Model file for the job. Use its own axes, mm. A direction names the side the tool comes from. Round coordinates to 2 decimals unless told otherwise and drop trailing zeros. Order: outer loops, then holes, each group sorted by start corner. A loop starts at its lowest first (then second) coordinate and runs counter-clockwise, first axis right, second up. Notation, with made-up numbers: (55, -33.5) - (59, -33.5) arc R13 cw to (59, -28.5) - close; hole circle Ø3 at (-30, -29). An arc over 180 degrees is marked (long way). Write item = value, one per line.
```python
from build123d import *

# Parameters (mm, degrees)
BOSS_EXTRUDE1_DEPTH                           = 2.54
CHAMFER1_SIZE                                 = 2.54
CSK_FOR_4_FLAT_HEAD_MACHINE_SCREW1_AT_2_COUNT = 2
CSK_FOR_4_FLAT_HEAD_MACHINE_SCREW1_AT_2_PITCH = 69.85
CSK_FOR_4_FLAT_HEAD_MACHINE_SCREW1_AT_3_COUNT = 2
CSK_FOR_4_FLAT_HEAD_MACHINE_SCREW1_AT_3_PITCH = 69.85
CSK_FOR_4_FLAT_HEAD_MACHINE_SCREW1_AT_4_COUNT = 2
CSK_FOR_4_FLAT_HEAD_MACHINE_SCREW1_AT_4_PITCH = 98.782817332
CUT_EXTRUDE2_DEPTH                            = 0.508


with BuildPart() as part:
    # Sketch1 → Boss-Extrude1 (new body)
    with BuildSketch(Plane(origin=(0, 0, 0), x_dir=(1, 0, 0), z_dir=(0, 1, 0))):
        with BuildLine():
            Line((-43.688, 34.925), (-43.688, -34.925))
            ThreePointArc((-43.688, -34.925), (-41.121376724, -41.121376724), (-34.925, -43.688))
            Line((-34.925, -43.688), (34.925, -43.688))
            ThreePointArc((34.925, -43.688), (41.121376724, -41.121376724), (43.688, -34.925))
            Line((43.688, -34.925), (43.688, 34.925))
            ThreePointArc((43.688, 34.925), (41.121376724, 41.121376724), (34.925, 43.688))
            Line((34.925, 43.688), (-34.925, 43.688))
            ThreePointArc((-34.925, 43.688), (-41.121376724, 41.121376724), (-43.688, 34.925))
        make_face()
    extrude(amount=BOSS_EXTRUDE1_DEPTH)

    # Chamfer1
    chamfer1_edges = [part.edges().sort_by_distance(p)[0] for p in [
        (-43.688, 0, 0),
        (-41.121376724, 0, 41.121376724),
        (-41.121376724, 0, -41.121376724),
        (0, 0, 43.688),
        (0, 0, -43.688),
        (41.121376724, 0, 41.121376724),
        (41.121376724, 0, -41.121376724),
        (43.688, 0, 0),
    ]]
    chamfer(chamfer1_edges, length=CHAMFER1_SIZE - 0.0001)  # a hair under: the kernel refuses the full size

    # Sketch6 → CSK for #4 Flat Head Machine Screw1 (revolve, cut)
    with BuildSketch(Plane(origin=(-34.925, 2.54, -34.925), x_dir=(0, 0, 1), z_dir=(1, 0, 0))):
        Polygon((0, 0), (0, 2.54), (1.7272, 2.54), (1.7272, 1.554265286), (3.0783022, 0), align=None)
    csk_for_4_flat_head_machine_screw1 = revolve(axis=Axis((-34.925, 8.89, -34.925), (0, -1, 0)), mode=Mode.SUBTRACT)

    # CSK for #4 Flat Head Machine Screw1 at 2: CSK for #4 Flat Head Machine Screw1 ×2
    with Locations(*[(i * CSK_FOR_4_FLAT_HEAD_MACHINE_SCREW1_AT_2_PITCH, 0, 0) for i in range(1, CSK_FOR_4_FLAT_HEAD_MACHINE_SCREW1_AT_2_COUNT)]):
        add(csk_for_4_flat_head_machine_screw1, mode=Mode.SUBTRACT)

    # CSK for #4 Flat Head Machine Screw1 at 3: CSK for #4 Flat Head Machine Screw1 ×2
    with Locations(*[(0, 0, i * CSK_FOR_4_FLAT_HEAD_MACHINE_SCREW1_AT_3_PITCH) for i in range(1, CSK_FOR_4_FLAT_HEAD_MACHINE_SCREW1_AT_3_COUNT)]):
        add(csk_for_4_flat_head_machine_screw1, mode=Mode.SUBTRACT)

    # CSK for #4 Flat Head Machine Screw1 at 4: CSK for #4 Flat Head Machine Screw1 ×2
    with Locations(*[Vector(0.7071067811865477, 0, 0.7071067811865475) * (i * CSK_FOR_4_FLAT_HEAD_MACHINE_SCREW1_AT_4_PITCH) for i in range(1, CSK_FOR_4_FLAT_HEAD_MACHINE_SCREW1_AT_4_COUNT)]):
        add(csk_for_4_flat_head_machine_screw1, mode=Mode.SUBTRACT)

    # Sketch3 → Cut-Extrude2 (cut)
    with BuildSketch(Plane(origin=(0, 2.54, 0), x_dir=(1, 0, 0), z_dir=(0, 1, 0))):
        Polygon((0, 3.81), (7.62, 3.81), (7.62, 9.525), (20.32, 0), (7.62, -9.525), (7.62, -3.81), (0, -3.81), (-20.32, -3.81), (-20.32, 3.81), align=None)
    extrude(amount=-CUT_EXTRUDE2_DEPTH, mode=Mode.SUBTRACT)


solid = part.part
```
1) Cut at B-B (y = 1.4). Write the cut outline in (x, z) (3 decimals), and give its area (3 significant figures).
Conclusion:
outline = (-42.548, -34.925) arc R7.623 ccw to (-34.925, -42.548) - (34.925, -42.548) arc R7.623 ccw to (42.548, -34.925) - (42.548, 34.925) arc R7.623 ccw to (34.925, 42.548) - (-34.925, 42.548) arc R7.623 ccw to (-42.548, 34.925) - close; hole circle Ø4.175 at (-34.925, -34.925); hole circle Ø4.175 at (-34.925, 34.925); hole circle Ø4.175 at (34.925, -34.925); hole circle Ø4.175 at (34.925, 34.925)
area = 7,140 mm^2
2) Wall check: line 1 along Z through (x, y) = (-34.5, 0.3); line 2 along X through (y, z) = (0.4, -35.5); line 3 along Z through (x, y) = (-36.5, 1.25). Give the ranges that are in metal, low to high.
Conclusion:
line_1 = -41.45 to -36.6, -33.25 to 33.25, 36.6 to 41.45
line_2 = -41.52 to -36.55, -33.3 to 33.3, 36.55 to 41.52
line_3 = -42.23 to -36.09, -33.76 to 33.76, 36.09 to 42.23
3) Flat gauge pins, fed straight in: pin 1 Ø5.5 at (x, z) = (-34.925, -34.925) entering from +Y; pin 2 Ø5.5 at (x, z) = (-0.5, 0.5) entering from +Y; pin 3 Ø1.5 at (x, y) = (-12.5, 1) entering from -Z. Where does each tip first touch, or does it go through?
Conclusion:
pin_1 = 2.16
pin_2 = 2.03
pin_3 = -42.9
4) Mould opens along X. For faces 3 (the face through (0.49, 1.25, -42.4)), 4 (the face through (-42.4, 1.25, -0.49)), 5 (the face through (36.7, 1.1, 34.5)) say: +X half, -X half, draft (parallel to the pull), parting line (faces both ways), or undercut.
Conclusion:
face_3 = draft
face_4 = -X half
face_5 = undercut
5) 3-axis set-ups, long thin cutter, end or side, ignore diameter. For faces 1 (the face through (14.059, 2.29, 4.696)), 2 (the face through (-36.638, 0.5, 34.7)): which of +Z, -Z, +X, -X, +Y, -Y reach the whole face in a straight line?
Conclusion:
face_1 = +Y
face_2 = +Y, -Y
